The model under review builds one solid part; all positions refer to its coordinate system, in mm. Round coordinates to 2 decimals unless told otherwise and drop trailing zeros. Order: outer loops, then holes, each group sorted by start corner. A loop starts at its lowest first (then second) coordinate and runs counter-clockwise, first axis right, second up. Notation, with made-up numbers: (-25.5, 10) -> (17.5, 10) arc R19 ccw to (17.5, 32) -> close; hole circle Ø3 at (69, 67.25). An arc over 180 degrees is marked (long way). Use a Markdown table: item, result. Add a question column.
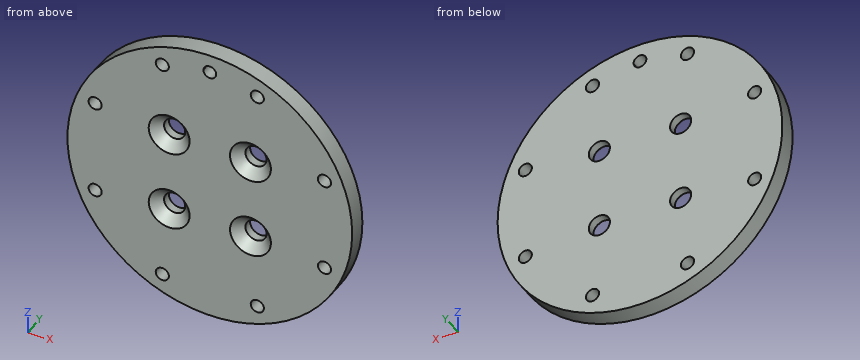
```python
from build123d import *

# Parameters (mm, degrees)
F0_R           = 39
F1_DEPTH       = 5
F3_D           = 3.6
F5_D           = 5.8
F5_CSINK_D     = 11.2
F5_CSINK_ANGLE = 90
F6_DEPTH       = 25


with BuildPart() as f1:
    # F0 (on Front) → F1 (new body)
    with BuildSketch(Plane.XZ):
        Circle(F0_R)
    extrude(amount=F1_DEPTH)

    # F3 (through all)
    with Locations(Plane.XZ.offset(5)):
        with Locations((31.4119041054, 13.0112367004), (13.0112367004, 31.4119041054), (-13.0112367004, 31.4119041054), (-31.4119041054, 13.0112367004), (-31.4119041054, -13.0112367004), (-13.0112367004, -31.4119041054), (13.0112367004, -31.4119041054), (31.4119041054, -13.0112367004)):
            Hole(F3_D / 2)

    # F5 (through all)
    with Locations(Plane.XZ.offset(5)):
        with Locations((11.1369318037, 11.1369318037), (-11.1369318037, 11.1369318037), (-11.1369318037, -11.1369318037), (11.1369318037, -11.1369318037)):
            CounterSinkHole(F5_D / 2, F5_CSINK_D / 2, counter_sink_angle=F5_CSINK_ANGLE)

    # F2 (on face) → F6 (cut)
    with BuildSketch(Plane.XZ.offset(5)):
        with BuildLine():
            ThreePointArc((-1.7494203868, 33.9549632353), (0, 32.25), (1.7494203868, 33.9549632353))
            ThreePointArc((1.7494203868, 33.9549632353), (0, 34), (-1.7494203868, 33.9549632353))
        make_face()
        with BuildLine():
            ThreePointArc((-1.7494203868, 33.9549632353), (0, 34), (1.7494203868, 33.9549632353))
            ThreePointArc((1.7494203868, 33.9549632353), (1.7498550907, 33.9774797529), (1.75, 34))
            ThreePointArc((1.75, 34), (-0.0225202471, 35.7498550907), (-1.7494203868, 33.9549632353))
        make_face()
    extrude(amount=-F6_DEPTH, mode=Mode.SUBTRACT)


solid = f1.part
```
Q1. Insertion check: pin 1 (1.5 mm diameter, centred on x = -31, z = 18, fed in from +Y); pin 2 (1 mm diameter, centred on y = -3, z = 1.5, fed in from -X); pin 3 (3 mm diameter, centred on x = -15, y = -3, fed in from +Z); pin 4 (1.5 mm diameter, centred on x = -21, y = -2.5, fed in from +Z). Each pin has a flat end and moves straight along its axis. Give the tip position at first contact, or say it passes through.
Q2. Add section A-A (y = -1.3). State how many separate pieces and enclosed holes the cut face has, then the cut area to 3 significant figures.
Q3. Add section C-C (z = 26). Write out the cut boundary in (x, y), then the cut area to 3 significant figures.
Q4. Wall thickness on line 1 (Z direction, x = 14, y = -2.85); line 2 (Z direction, x = 32, y = -2.8); line 3 (X direction, y = -1.1, z = 31.5): over which ranges is each line inside the solid? List them lowest first. Write a range as [from, to].
Q5. Add section B-B (z = -27.5). Write out the cut boundary in (x, y).
Report:
| question | item | result |
|---|---|---|
| 1 | pin 1 | stops at y = 0 |
| 1 | pin 2 | stops at x = -38.99 |
| 1 | pin 3 | stops at z = 36.59 |
| 1 | pin 4 | stops at z = 33.33 |
| 2 | separate pieces | 1 |
| 2 | enclosed holes | 13 |
| 2 | area | 4,580 mm² |
| 3 | outline | (-29.07, -5) -> (29.07, -5) -> (29.07, 0) -> (-29.07, 0) -> close |
| 3 | area | 291 mm² |
| 4 | line 1 | z = [-36.4, -32.92], [-29.91, -13.06], [-9.21, 9.21], [13.06, 29.91], [32.92, 36.4] |
| 4 | line 2 | z = [-22.29, -14.71], [-11.31, 11.31], [14.71, 22.29] |
| 4 | line 3 | x = [-22.99, -14.81], [-11.21, 11.21], [14.81, 22.99] |
| 5 | outline | (-27.65, -5) -> (27.65, -5) -> (27.65, 0) -> (-27.65, 0) -> close |
